Geometry: final body of the model. Coordinates: model frame, mm. A direction names the side the tool comes from. Give positions to 0.01 mm unless a question says otherwise; leave off trailing zeros. Order: outer loops, then holes, each group sorted by start corner. A loop starts at its lowest first (then second) coordinate and runs counter-clockwise, first axis right, second up. Notation, with made-up numbers: (89.5, 47.25) - (99.5, 47.25) arc R12 cw to (99.5, 52.25) - close; hole circle Ø2 at (83.25, 73). An arc over 180 degrees is marked (long way). Write item = value, one per line. Start each with the question number.
from build123d import *

# Parameters (mm, degrees)
SKETCH1_W           = 44.4
SKETCH1_H           = 40
SKETCH1_R           = 2.1
BOSS_EXTRUDE1_DEPTH = 2
SKETCH2_W           = 44.4
SKETCH2_H           = 18.3
BOSS_EXTRUDE2_DEPTH = 2
LPATTERN1_COUNT     = 2
LPATTERN1_PITCH     = 16.3
SKETCH3_R           = 2.15
CUT_EXTRUDE1_DEPTH  = 64.253853638
FILLET4_R           = 1


with BuildPart() as part:
    # Sketch1 → Boss-Extrude1 (new body)
    with BuildSketch(Plane.XY):
        with Locations((22.2, 20)):
            Rectangle(SKETCH1_W, SKETCH1_H)
        with Locations((8, 8.476902454)):
            Circle(SKETCH1_R, mode=Mode.SUBTRACT)
        with Locations((8, 29.976902454)):
            Circle(SKETCH1_R, mode=Mode.SUBTRACT)
        with Locations((36.4, 29.976902454)):
            Circle(SKETCH1_R, mode=Mode.SUBTRACT)
        with Locations((36.4, 8.476902454)):
            Circle(SKETCH1_R, mode=Mode.SUBTRACT)
    boss_extrude1 = extrude(amount=BOSS_EXTRUDE1_DEPTH)

    # Sketch2 → Boss-Extrude2 (add)
    with BuildSketch(Plane(origin=(0, 40, 0), x_dir=(1, 0, 0), z_dir=(0, 1, 0))):
        with Locations((22.2, 7.15)):
            Rectangle(SKETCH2_W, SKETCH2_H)
    extrude(amount=BOSS_EXTRUDE2_DEPTH)

    # LPattern1: Boss-Extrude1 ×2
    with Locations(*[(0, 0, -i * LPATTERN1_PITCH) for i in range(1, LPATTERN1_COUNT)]):
        add(boss_extrude1)

    # Sketch3 → Cut-Extrude1 (cut, through all)
    with BuildSketch(Plane(origin=(0, 42, 0), x_dir=(1, 0, 0), z_dir=(0, 1, 0))):
        with Locations(Location((12.2, 7.15, 0), (0, 0, 270))):
            Circle(SKETCH3_R)
        with Locations(Location((32.2, 7.15, 0), (0, 0, 270))):
            Circle(SKETCH3_R)
    extrude(amount=-CUT_EXTRUDE1_DEPTH, mode=Mode.SUBTRACT)

    # Fillet4
    fillet4_edges = [part.edges().sort_by_distance(p)[0] for p in [
        (44.4, 21, 2),
        (0, 21, -16.3),
        (44.4, 21, -16.3),
        (0, 42, -7.15),
        (22.2, 42, 2),
        (44.4, 42, -7.15),
        (22.2, 42, -16.3),
        (22.2, 40, -14.3),
        (22.2, 0, -16.3),
        (0, 0, -15.3),
        (44.4, 0, -15.3),
        (0, 21, 2),
        (22.2, 40, 0),
        (44.4, 0, 1),
        (0, 0, 1),
        (22.2, 0, 2),
    ]]
    fillet(fillet4_edges, radius=FILLET4_R)


solid = part.part
Q1. Pull-direction query (Z, two-part tool) for faces 1 (the flat face through (22, 21, 2)), 2 (the cylindrical face through (0.285, 41.699, -7.264)), 3 (the cylindrical face through (22.511, 39.699, -14.015)); classes: +Z half, -Z half, draft (parallel to the pull), parting line (faces both ways), or undercut.
Q2. Section A-A, the plane x = 32.2. Return the cut outline in (y, z).
Q3. Section D-D, the plane x = 9.5. Count the separate pieces of the cut face and the enclosed holes in it, then the cut area to 3 significant figures.
Q4. Set-up query: faces 4 (the cylindrical face through (22.511, 39.715, -0.301)), 5 (the cylindrical face through (37.369, 6.614, 0.986)). Return all of +Z, -Z, +X, -X, +Y, -Y with unobstructed straight access to the full face (end or side cutting, diameter ignored); none if empty.
Q5. Section B-B, the plane y = 3.5. Return the cut outline in (x, z), then the cut area to 3 significant figures.
Q6. Section C-C, the plane z = -11. Return the cut outline in (x, y).
Q7. Contact query for flat-ended pins moving along their axis: pin 1 (3.5 mm diameter, centred on x = 8, y = 29.98, fed in from +Z); pin 2 (7 mm diameter, centred on x = 32.2, z = -7.15, fed in from -Y); pin 3 (5.5 mm diameter, centred on x = 36.4, y = 8.48, fed in from +Z). Output: stop coordinate, or through.
Q8. Material intervals for line 1 along Y through (x, z) = (8, 1.15); line 2 along Z through (x, y) = (40.5, 34); line 3 along X through (y, z) = (7.5, 0.25), sorted ascending. Write a range as from..to.
The answers:
q1.face_1 = +Z half
q1.face_2 = draft
q1.face_3 = undercut
q2.outline = (0, -15.3) arc R1 ccw to (1, -16.3) - (41, -16.3) arc R1 ccw to (42, -15.3) - (42, -9.3) - (40, -9.3) - (40, -13.3) arc R1 cw to (39, -14.3) - (0, -14.3) - close; (0, 0) - (39, 0) arc R1 cw to (40, -1) - (40, -5) - (42, -5) - (42, 1) arc R1 ccw to (41, 2) - (1, 2) arc R1 ccw to (0, 1) - close
q3.separate_pieces = 5
q3.enclosed_holes = 0
q3.area = 173 mm²
q4.face_4 = +X, -X, -Y
q4.face_5 = +Z, -Z
q5.outline = (0, -15.3) arc R1 ccw to (1, -16.3) - (43.4, -16.3) arc R1 ccw to (44.4, -15.3) - (44.4, -14.3) - (0, -14.3) - close; (0, 0) - (44.4, 0) - (44.4, 1) arc R1 ccw to (43.4, 2) - (1, 2) arc R1 ccw to (0, 1) - close
q5.area = 177 mm²
q6.outline = (0, 40) - (44.4, 40) - (44.4, 41) arc R1 ccw to (43.4, 42) - (1, 42) arc R1 ccw to (0, 41) - close
q7.pin_1 = through
q7.pin_2 = 40
q7.pin_3 = 2
q8.line_1 = 0.01..6.38, 10.58..27.88, 32.08..41.99
q8.line_2 = -16.3..-14.3, 0..2
q8.line_3 = 0..6.14, 9.86..34.54, 38.26..44.4
